Design review of the part built by this model. Coordinates are the model's own, in mm. A direction names the side the tool comes from. Give positions to 0.01 mm unless a question says otherwise; leave off trailing zeros. Write each loop counter-clockwise with the first axis right and the second up, starting at its lowest first coordinate (ties: lowest second). Pieces come first, ordered by that corner, then holes. Notation, with made-up numbers: (-18.5, 2) - (35.5, 2) arc R8 ccw to (35.5, 16) - close; hole circle Ø11 at (-36, -17). An arc over 180 degrees is marked (long way). Use a Markdown table: item, result. Add a question column.
```python
from build123d import *

# Parameters (mm, degrees)
F0_R     = 1.27
F1_DEPTH = 9.525
F2_DEPTH = 6.35


with BuildPart() as f1:
    # F0 (on Right) → F1 (new body, symmetric)
    with BuildSketch(Plane.YZ):
        with BuildLine():
            ThreePointArc((-7.199729, 6.236147), (-3.327777, -8.92477), (9.525, 0))
            ThreePointArc((9.525, 0), (8.919603, 3.341602), (7.180369, 6.258429))
            ThreePointArc((7.180369, 6.258429), (-0.014759, 9.524989), (-7.199729, 6.236147))
        make_face()
        Circle(F0_R, mode=Mode.SUBTRACT)
    extrude(amount=F1_DEPTH, both=True)

    # F0 (on Right) → F2 (join, symmetric)
    with BuildSketch(Plane.YZ):
        with BuildLine():
            ThreePointArc((-7.199729, 6.236147), (-0.014759, 9.524989), (7.180369, 6.258429))
            Line((7.180369, 6.258429), (13.829825, 23.957072))
            Line((13.829825, 23.957072), (17.903983, 34.801126))
            Line((17.903983, 34.801126), (-18.993251, 75.119182))
            Line((-18.993251, 75.119182), (-56.423347, 63.391089))
            Line((-56.423347, 63.391089), (-41.950375, 60.147148))
            Line((-41.950375, 60.147148), (-38.207367, 63.391089))
            Line((-38.207367, 63.391089), (-36.728468, 58.671199))
            Line((-36.728468, 58.671199), (-33.208895, 61.61258))
            Line((-33.208895, 61.61258), (-31.90448, 57.449549))
            Line((-31.90448, 57.449549), (-28.797716, 60.147148))
            Line((-28.797716, 60.147148), (-27.610865, 56.359325))
            Line((-27.610865, 56.359325), (-24.386536, 58.789425))
            Line((-24.386536, 58.789425), (-23.207981, 55.028077))
            Line((-23.207981, 55.028077), (-19.397542, 44.635847))
            Line((-19.397542, 44.635847), (-7.199729, 6.236147))
        make_face()
        Polygon((-30.50116, 66.842455), (-19.397542, 70.495695), (-16.252705, 61.489249), align=None, mode=Mode.SUBTRACT)
        Polygon((0, 14.982579), (-10.09386, 45.661755), (-13.11075, 55.028077), (6.752282, 32.954909), align=None, mode=Mode.SUBTRACT)
    extrude(amount=F2_DEPTH, both=True)


solid = f1.part
```
(1) Add section A-A (z = 17.5). State the section outline as (x, y) points.
(2) Mouldability with a two-part tool opening along Z and no side actions: class faces 4 (the face through (0.089, -13.384, 25.705)), 5 (the face through (-6.35, -11, 43)), 6 (the face through (0.089, -21.329, 49.905)) as +Z half, -Z half, draft (parallel to the pull), parting line (faces both ways), or undercut.
(3) Add section C-C (y = -18). State the section outline as (x, z) points, and give its area (3 significant figures).
(4) For line 1 along Y through (x, z) = (-4.5, 17); line 2 along X through (y, z) = (8, 12.5); line 3 along Y through (x, z) = (-5.5, 56.5), list the stretches that pass through material, from the lowest coordinate up.
(5) Tool access review of faces 1 (the face through (0.089, -49.288, 61.792)), 2 (the face through (0.089, -28.213, 58.28)), 3 (the face through (0.09, -17.85, 66.06)): name each direction out of +Z, -Z, +X, -X, +Y, -Y from which nothing blocks a thin tool from reaching the whole face with its end or side.
(6) Insertion check: pin 1 (2 mm diameter, centred on x = -5, y = -41, fed in from +Z); pin 2 (10 mm diameter, centred on x = 3.5, z = 2.5, fed in from -Y) (3 decimals); pin 3 (12 mm diameter, centred on y = -10.5, z = 27.5, fed in from -X). Each pin has a flat end and moves straight along its axis. Give the tip position at first contact, or say it passes through.
(7) Add section B-B (x = -1.75). State the section outline as (y, z) points (3 decimals), and give its area (3 significant figures).
Answers follow:
| question | item | result |
|---|---|---|
| 1 | outline | (-6.35, -10.78) - (6.35, -10.78) - (6.35, -0.83) - (-6.35, -0.83) - close; (-6.35, 0.95) - (6.35, 0.95) - (6.35, 11.4) - (-6.35, 11.4) - close |
| 2 | face 4 | undercut |
| 2 | face 5 | draft |
| 2 | face 6 | -Z half |
| 3 | outline | (-6.35, 40.24) - (6.35, 40.24) - (6.35, 62.15) - (-6.35, 62.15) - close; (-6.35, 66.49) - (6.35, 66.49) - (6.35, 74.03) - (-6.35, 74.03) - close |
| 3 | area | 374 mm^2 |
| 4 | line 1 | -10.62 to -0.66, 0.76 to 11.22 |
| 4 | line 2 | -6.35 to 6.35 |
| 4 | line 3 | -27.65 to -27.42, -23.67 to -1.95 |
| 5 | face 1 | -Z, +X, -X, -Y |
| 5 | face 2 | -Z, +X, -X |
| 5 | face 3 | +X, -X |
| 6 | pin 1 | z = 68.54 |
| 6 | pin 2 | y = -9.525 |
| 6 | pin 3 | x = -6.35 |
| 7 | outline | (-56.423, 63.391) - (-41.95, 60.147) - (-38.207, 63.391) - (-36.728, 58.671) - (-33.209, 61.613) - (-31.904, 57.45) - (-28.798, 60.147) - (-27.611, 56.359) - (-24.387, 58.789) - (-23.208, 55.028) - (-19.398, 44.636) - (-7.2, 6.236) arc R9.525 ccw (long way) to (9.525, 0) arc R9.525 ccw to (7.18, 6.258) - (17.904, 34.801) - (-18.993, 75.119) - close; hole (-30.501, 66.842) - (-16.253, 61.489) - (-19.398, 70.496) - close; hole (-13.111, 55.028) - (-10.094, 45.662) - (0, 14.983) - (6.752, 32.955) - close; hole circle Ø2.54 at (0, 0) |
| 7 | area | 1,740 mm^2 |
